The listing builds one solid part. Answer for the finished solid, in the listing's coordinates (mm). Give positions to 0.01 mm unless a question says otherwise; leave off trailing zeros. Write each loop counter-clockwise with the first axis right and the second up, starting at its lowest first coordinate (ties: lowest second). Pieces come first, ordered by that corner, then holes. Notation, with made-up numbers: (1.25, 44.5) - (46.25, 44.5) arc R30 cw to (46.25, 76.5) - close; hole circle Ø9 at (-12.75, 86.5). An arc over 180 degrees is marked (long way). Use a Markdown table: item, result. Add a question column.
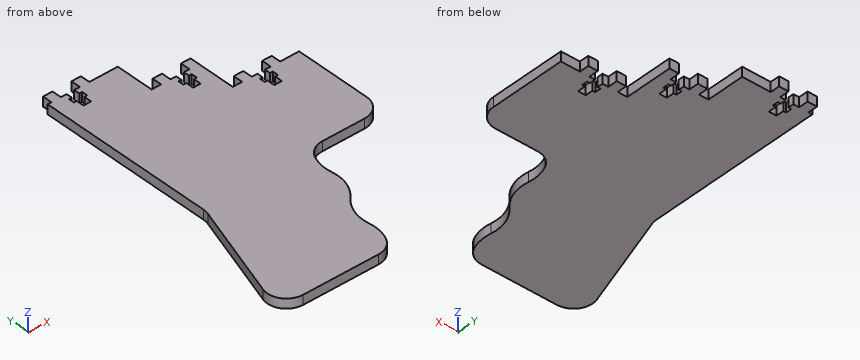
from build123d import *

# Parameters (mm, degrees)
BOSS_EXTRU_1_DEPTH = 5
CONG_1_R           = 10


with BuildPart() as part:
    # Esquisse1 → Boss.-Extru.1 (new body)
    with BuildSketch(Plane.XY):
        with BuildLine():
            Line((10, 0), (10, -20))
            Line((10, -20), (15, -20))
            Line((15, -20), (15, -15))
            Line((15, -15), (20, -15))
            Line((20, -15), (20, -20))
            Line((20, -20), (23, -20))
            Line((23, -20), (23, -23))
            Line((23, -23), (21.5, -23))
            Line((21.5, -23), (21.5, -26))
            Line((21.5, -26), (23, -26))
            Line((23, -26), (23, -30))
            Line((23, -30), (27, -30))
            Line((27, -30), (27, -26))
            Line((27, -26), (28.5, -26))
            Line((28.5, -26), (28.5, -23))
            Line((28.5, -23), (27, -23))
            Line((27, -23), (27, -20))
            Line((27, -20), (30, -20))
            Line((30, -20), (30, -15))
            Line((30, -15), (35, -15))
            Line((35, -15), (35, -20))
            Line((35, -20), (45, -20))
            Line((45, -20), (45, -70))
            Line((45, -70), (7.744378736, -70))
            ThreePointArc((7.744378736, -70), (2.794303084, -78.065385001), (2.058284052, -87.5))
            ThreePointArc((2.058284052, -87.5), (1.322265021, -96.934614999), (-3.627810632, -105))
            ThreePointArc((-3.627810632, -105), (-8.577886284, -113.065385001), (-9.313905316, -122.5))
            ThreePointArc((-9.313905316, -122.5), (-10.049924347, -131.934614999), (-15, -140))
            Line((-15, -140), (-73.488757473, -140))
            Line((-73.488757473, -140), (-52, -73.864404892))
            Line((-52, -73.864404892), (-52, 20))
            Line((-52, 20), (-50, 20))
            Line((-50, 20), (-50, 25))
            Line((-50, 25), (-45, 25))
            Line((-45, 25), (-45, 20))
            Line((-45, 20), (-42, 20))
            Line((-42, 20), (-42, 17))
            Line((-42, 17), (-43.5, 17))
            Line((-43.5, 17), (-43.5, 14))
            Line((-43.5, 14), (-42, 14))
            Line((-42, 14), (-42, 10))
            Line((-42, 10), (-38, 10))
            Line((-38, 10), (-38, 14))
            Line((-38, 14), (-36.5, 14))
            Line((-36.5, 14), (-36.5, 17))
            Line((-36.5, 17), (-38, 17))
            Line((-38, 17), (-38, 20))
            Line((-38, 20), (-35, 20))
            Line((-35, 20), (-35, 25))
            Line((-35, 25), (-30, 25))
            Line((-30, 25), (-30, 20))
            Line((-30, 20), (-15, 20))
            Line((-15, 20), (-15, 0))
            Line((-15, 0), (-10, 0))
            Line((-10, 0), (-10, 5))
            Line((-10, 5), (-5, 5))
            Line((-5, 5), (-5, 0))
            Line((-5, 0), (-2, 0))
            Line((-2, 0), (-2, -3))
            Line((-2, -3), (-3.5, -3))
            Line((-3.5, -3), (-3.5, -6))
            Line((-3.5, -6), (-2, -6))
            Line((-2, -6), (-2, -10))
            Line((-2, -10), (2, -10))
            Line((2, -10), (2, -6))
            Line((2, -6), (3.5, -6))
            Line((3.5, -6), (3.5, -3))
            Line((3.5, -3), (2, -3))
            Line((2, -3), (2, 0))
            Line((2, 0), (5, 0))
            Line((5, 0), (5, 5))
            Line((5, 5), (10, 5))
            Line((10, 5), (10, 0))
        make_face()
    extrude(amount=BOSS_EXTRU_1_DEPTH)

    # Congé1
    cong_1_edges = [part.edges().sort_by_distance(p)[0] for p in [
        (45, -70, 2.5),
        (7.744378736, -70, 2.5),
        (-15, -140, 2.5),
        (-73.488757473, -140, 2.5),
        (-52, -73.864404892, 2.5),
    ]]
    fillet(cong_1_edges, radius=CONG_1_R)


solid = part.part
1. The part is cut by section A-A (y = -33.5). Give the vertices of the cut face in (x, z).
2. The part is cut by section B-B (y = -102). Give the vertices of the cut face in (x, z), and give its area (3 significant figures).
3. Consider L1, parallel to X at y = -29, z = 0.4; L2, parallel to Y at x = -29, z = 0.25; L3, parallel to Y at x = 26, z = 3.7. Determine where each line is inside the solid, lowest interval first. Write a range as [from, to].
4. Given P1, Ø1.2, axis at y = 11, z = 1.5, coming from the +X side; P2, Ø2.5, axis at y = 23.5, z = 2, coming from the -X side; P3, Ø1.5, axis at y = -1, z = 3, coming from the -X side; P4, Ø4, axis at x = -38, y = -16.5, coming from the -Z side, each flat-ended and moving along its own axis, determine where each tip first touches the part or whether it passes through.
Check values:
| question | item | result |
|---|---|---|
| 1 | outline | (-52, 0) - (45, 0) - (45, 5) - (-52, 5) - close |
| 2 | outline | (-61.14, 0) - (-1.15, 0) - (-1.15, 5) - (-61.14, 5) - close |
| 2 | area | 300 mm2 |
| 3 | L1 | x = [-52, 23], [27, 45] |
| 3 | L2 | y = [-140, 20] |
| 3 | L3 | y = [-70, -30] |
| 4 | P1 | stops at x = -15 |
| 4 | P2 | stops at x = -50 |
| 4 | P3 | stops at x = -52 |
| 4 | P4 | stops at z = 0 |
